Could you check a few things on this model? Use its own coordinates, in mm. Give positions to 0.01 mm unless a question says otherwise; leave off trailing zeros. Loops run counter-clockwise (first coordinate to the right, second up) from the corner with the lowest first, then second, coordinate; pieces in that order, holes last. Notation, with made-up numbers: M 16,4 L 63,4 A19 ccw 63,35 Z; hole C 74,37.5 d2. An arc over 180 degrees is marked long. Answer in a Markdown table with one row per item. Add a question column.
1. If we section it at A-A on x = -350: List the corners of the cut face in (y, z) for me, then the cut area to 3 significant figures.
2. If we section it at C-C on z = 7.75: Count the separate pieces of the cut face and the enclosed holes in it, then the cut area to 3 significant figures.
3. If we section it at B-B on y = 370: List the corners of the cut face in (x, z) for me.
4. I need wall thicknesses on line 1 along Y through (x, z) = (-350, 5.5); line 2 along Y through (x, z) = (-257, 13). Which ranges of each line are inside material? Lowest first, please. Write a range as from..to.
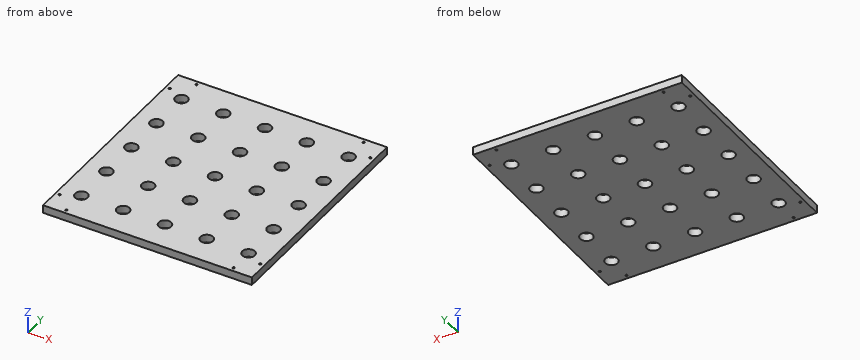
```python
from build123d import *

# Parameters (mm, degrees)
SKETCH_W      = 500
SKETCH_H      = 540
SKETCH_R      = 15
SKETCH_R_2    = 2.5
EXTRUDE_DEPTH = 19


with BuildPart() as part:
    # Sketch → Extrude (new body)
    with BuildSketch(Plane.XY):
        with Locations((-250, 270)):
            Rectangle(SKETCH_W, SKETCH_H)
        with Locations((-450, 470)):
            Circle(SKETCH_R, mode=Mode.SUBTRACT)
        with Locations((-350, 470)):
            Circle(SKETCH_R, mode=Mode.SUBTRACT)
        with Locations((-250, 470)):
            Circle(SKETCH_R, mode=Mode.SUBTRACT)
        with Locations((-150, 470)):
            Circle(SKETCH_R, mode=Mode.SUBTRACT)
        with Locations((-50, 470)):
            Circle(SKETCH_R, mode=Mode.SUBTRACT)
        with Locations((-450, 370)):
            Circle(SKETCH_R, mode=Mode.SUBTRACT)
        with Locations((-450, 270)):
            Circle(SKETCH_R, mode=Mode.SUBTRACT)
        with Locations((-450, 170)):
            Circle(SKETCH_R, mode=Mode.SUBTRACT)
        with Locations((-450, 70)):
            Circle(SKETCH_R, mode=Mode.SUBTRACT)
        with Locations((-350, 370)):
            Circle(SKETCH_R, mode=Mode.SUBTRACT)
        with Locations((-250, 370)):
            Circle(SKETCH_R, mode=Mode.SUBTRACT)
        with Locations((-150, 370)):
            Circle(SKETCH_R, mode=Mode.SUBTRACT)
        with Locations((-50, 370)):
            Circle(SKETCH_R, mode=Mode.SUBTRACT)
        with Locations((-350, 270)):
            Circle(SKETCH_R, mode=Mode.SUBTRACT)
        with Locations((-250, 270)):
            Circle(SKETCH_R, mode=Mode.SUBTRACT)
        with Locations((-150, 270)):
            Circle(SKETCH_R, mode=Mode.SUBTRACT)
        with Locations((-50, 270)):
            Circle(SKETCH_R, mode=Mode.SUBTRACT)
        with Locations((-350, 170)):
            Circle(SKETCH_R, mode=Mode.SUBTRACT)
        with Locations((-250, 170)):
            Circle(SKETCH_R, mode=Mode.SUBTRACT)
        with Locations((-150, 170)):
            Circle(SKETCH_R, mode=Mode.SUBTRACT)
        with Locations((-50, 170)):
            Circle(SKETCH_R, mode=Mode.SUBTRACT)
        with Locations((-350, 70)):
            Circle(SKETCH_R, mode=Mode.SUBTRACT)
        with Locations((-250, 70)):
            Circle(SKETCH_R, mode=Mode.SUBTRACT)
        with Locations((-150, 70)):
            Circle(SKETCH_R, mode=Mode.SUBTRACT)
        with Locations((-50, 70)):
            Circle(SKETCH_R, mode=Mode.SUBTRACT)
        with Locations((-450, 530)):
            Circle(SKETCH_R_2, mode=Mode.SUBTRACT)
        with Locations((-490, 490)):
            Circle(SKETCH_R_2, mode=Mode.SUBTRACT)
        with Locations((-50, 530)):
            Circle(SKETCH_R_2, mode=Mode.SUBTRACT)
        with Locations((-10, 490)):
            Circle(SKETCH_R_2, mode=Mode.SUBTRACT)
        with Locations((-490, 50)):
            Circle(SKETCH_R_2, mode=Mode.SUBTRACT)
        with Locations((-450, 10)):
            Circle(SKETCH_R_2, mode=Mode.SUBTRACT)
        with Locations((-10, 50)):
            Circle(SKETCH_R_2, mode=Mode.SUBTRACT)
        with Locations((-50, 10)):
            Circle(SKETCH_R_2, mode=Mode.SUBTRACT)
    extrude(amount=EXTRUDE_DEPTH)


solid = part.part
```
Results:
| question | item | result |
|---|---|---|
| 1 | outline | M 0,0 L 55,0 L 55,19 L 0,19 Z; M 85,0 L 155,0 L 155,19 L 85,19 Z; M 185,0 L 255,0 L 255,19 L 185,19 Z; M 285,0 L 355,0 L 355,19 L 285,19 Z; M 385,0 L 455,0 L 455,19 L 385,19 Z; M 485,0 L 540,0 L 540,19 L 485,19 Z |
| 1 | area | 7,410 mm2 |
| 2 | separate pieces | 1 |
| 2 | enclosed holes | 33 |
| 2 | area | 252,000 mm2 |
| 3 | outline | M -500,0 L -465,0 L -465,19 L -500,19 Z; M -435,0 L -365,0 L -365,19 L -435,19 Z; M -335,0 L -265,0 L -265,19 L -335,19 Z; M -235,0 L -165,0 L -165,19 L -235,19 Z; M -135,0 L -65,0 L -65,19 L -135,19 Z; M -35,0 L 0,0 L 0,19 L -35,19 Z |
| 4 | line 1 | 0..55, 85..155, 185..255, 285..355, 385..455, 485..540 |
| 4 | line 2 | 0..56.73, 83.27..156.73, 183.27..256.73, 283.27..356.73, 383.27..456.73, 483.27..540 |
